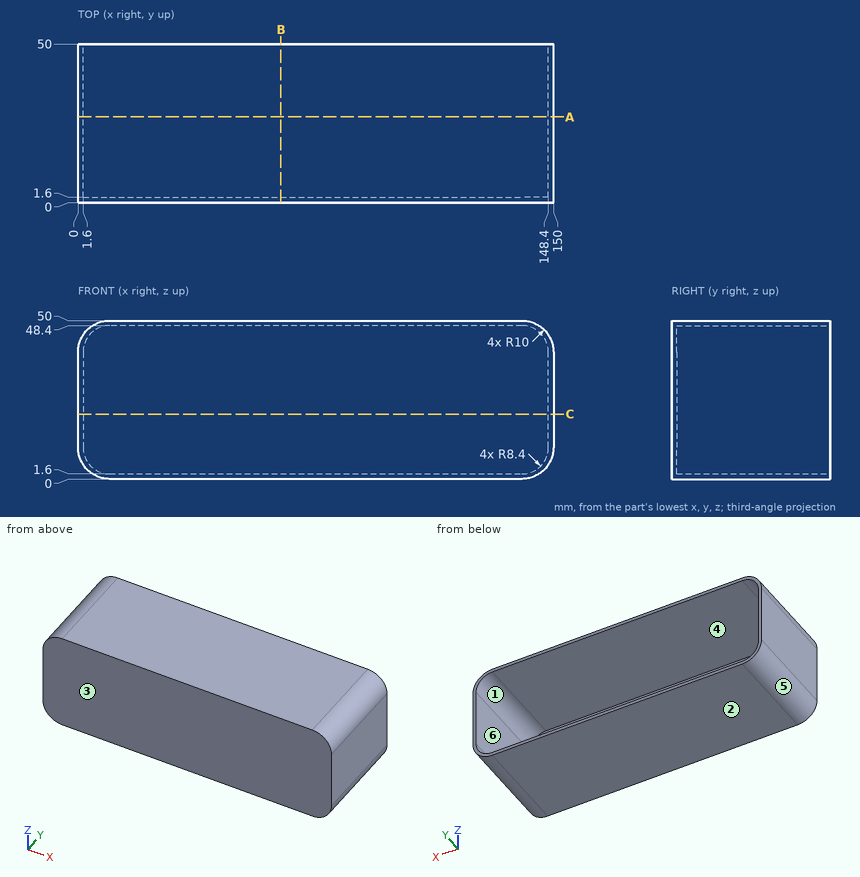
Job drawing, mm, ordinate dimensions from the low corner. One solid piece. A direction names the side the tool comes from. Give positions to 0.01 mm unless a question says otherwise; leave off trailing zeros. Loops run counter-clockwise (first coordinate to the right, second up) from the corner with the lowest first, then second, coordinate; pieces in that order, holes last. Notation, with made-up numbers: (33.5, -39) - (41.5, -39) arc R23 ccw to (41.5, -27) - close; hole circle Ø10 at (-15.75, -7). An arc over 180 degrees is marked (long way). Use one line per item in the form item = value.
(1) Cut at C-C (z = 20.5). Give the cut face in (x, y), then the cut area to 3 significant figures.
Determined:
outline = (0, 0) - (150, 0) - (150, 50) - (148.4, 50) - (148.4, 1.6) - (1.6, 1.6) - (1.6, 50) - (0, 50) - close
area = 395 mm^2
(2) Drill centre lines: L1, parallel to X at y = 12, z = 12; L2, parallel to Z at x = 13.5, y = 4; L3, parallel to Y at x = 55.5, z = 37. Where is each one in solid material? Low to high.
Determined:
L1 = 0 to 1.6, 148.4 to 150
L2 = 0 to 1.6, 48.4 to 50
L3 = 0 to 1.6
(3) Cut at A-A (y = 27). Give the cut face in (x, z), then the cut area to 3 significant figures.
Determined:
outline = (0, 10) arc R10 ccw to (10, 0) - (140, 0) arc R10 ccw to (150, 10) - (150, 40) arc R10 ccw to (140, 50) - (10, 50) arc R10 ccw to (0, 40) - close; hole (1.6, 10) arc R8.4 ccw to (10, 1.6) - (140, 1.6) arc R8.4 ccw to (148.4, 10) - (148.4, 40) arc R8.4 ccw to (140, 48.4) - (10, 48.4) arc R8.4 ccw to (1.6, 40) - close
area = 604 mm^2
(4) Cut at B-B (x = 64). Give the cut face in (y, z), then the cut area to 3 significant figures.
Determined:
outline = (0, 0) - (50, 0) - (50, 1.6) - (1.6, 1.6) - (1.6, 48.4) - (50, 48.4) - (50, 50) - (0, 50) - close
area = 235 mm^2
(5) Pull direction Z, two halves, no side cores. Call the marked faces 1, 2, 3 and 4: pulls with the +Z half, pulls with the -Z half, needs draft (parallel to the pull), parting line crosses it, or undercut.
Determined:
face_1 = undercut
face_2 = pulls with the -Z half
face_3 = needs draft
face_4 = undercut
(6) 3-axis set-ups, long thin cutter, end or side, ignore diameter. For the marked faces 5 and 6: which of +Z, -Z, +X, -X, +Y, -Y reach the whole face in a straight line?
Determined:
face_5 = -Z, -X, +Y, -Y
face_6 = +Y
(7) Drop a flat-ended pin along its axis: P1, Ø23.5, axis at x = 91.5, z = 31.5, coming from the +Y side. Give the stop position or say it passes through.
Determined:
P1 = 1.6
